from build123d import *

# Parameters (mm, degrees)
F1_DEPTH = 3
F2_ANGLE = 30


with BuildPart() as f1:
    # F0 (on Top) → F1 (new body)
    with BuildSketch(Plane.XY):
        Polygon((-92.6405740249, -53.4860603511), (92.6405740249, -53.4860603511), (69.4804305186, -13.3715150878), (173.2050807569, 46.5139396489), (289.0674983355, 113.4071376268), (285.7992481602, 119.0679129823), (242.747211323, 193.6362281535), (126.8847937445, 126.7430301756), (23.1601435062, 66.8575754389), (0, 106.9721207023), align=None)
    extrude(amount=F1_DEPTH)


with BuildPart() as f1_1:
    # F2: moved
    add(f1.part.rotate(Axis((92.6405740249, -53.4860603511, 1.5), (0, 0, -1)), F2_ANGLE))


solid = f1_1.part
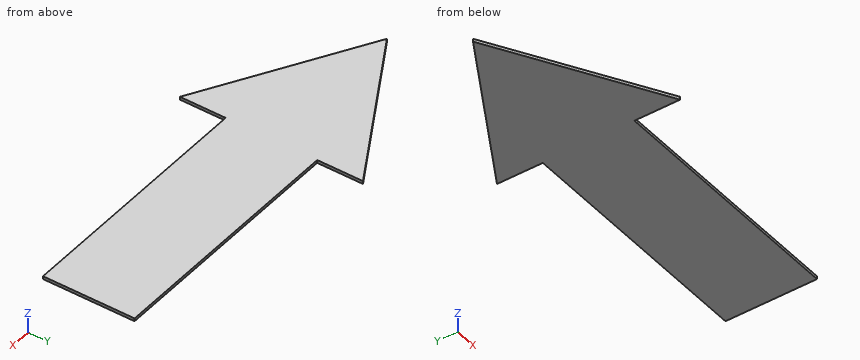
The listing builds one solid part. Answer for the finished solid, in the listing's coordinates (mm). Coordinates: 2 decimals unless noted, no trailing zeros. Write each loop counter-clockwise with the first axis right and the second up, starting at its lowest first coordinate (ties: lowest second). Pieces come first, ordered by that corner, then holes. Notation, with made-up numbers: (-6.5, 3.25) - (16.5, 3.25) arc R19 cw to (16.5, 16.25) - close; hole circle Ø5 at (-27, 57.5). An arc over 180 degrees is marked (long way). Return JSON: item names as keys, results as strings.
1. Consider line 1 along Y through (x, z) = (149, 2.3); line 2 along X through (y, z) = (-30, 1.5); line 3 along X through (y, z) = (87, 2.2). Determine where each line is inside the solid, lowest interval first.
Final values:
{"line 1": "-7.17 to 85.47", "line 2": "51.96 to 92.64", "line 3": "15.05 to 92.64"}
2. Each of these flat-tipped pins is pushed along its axis until it touches: pin 1 Ø1 at (x, z) = (85, 2.5) entering from +Y; pin 2 Ø1.5 at (y, z) = (104, 1.5) entering from +X; pin 3 Ø1.5 at (x, z) = (110.5, 1.5) entering from +Y. Where does it stop, or does it pass through?
Final values:
{"pin 1": "y = 127.67", "pin 2": "x = 92.64", "pin 3": "y = 85.47"}
3. The part is cut by section A-A on z = 1.05. Determine the outline of the cut face in (x, y).
Final values:
{"outline": "(-67.82, 39.15) - (92.64, -53.49) - (92.64, -7.17) - (346.2, -7.17) - (346.2, 85.47) - (92.64, 85.47) - (92.64, 131.8) - close"}
4. The part is cut by section C-C on y = 112. Determine the outline of the cut face in (x, z), then the cut area to 3 significant figures.
Final values:
{"outline": "(58.35, 0) - (92.64, 0) - (92.64, 3) - (58.35, 3) - close", "area": "103 mm^2"}
5. The part is cut by section B-B on x = 191.5. Determine the outline of the cut face in (y, z).
Final values:
{"outline": "(-7.17, 0) - (85.47, 0) - (85.47, 3) - (-7.17, 3) - close"}
